Geometry check sheet. Reference: the model listing, model coordinates, mm. A direction names the side the tool comes from. Coordinates: 2 decimals unless noted, no trailing zeros. Loops run counter-clockwise (first coordinate to the right, second up) from the corner with the lowest first, then second, coordinate; pieces in that order, holes last.
from build123d import *

# Parameters (mm, degrees)
F1_DEPTH = 25.4
F3_D     = 5.1054
F4_R     = 6.35
F5_DEPTH = 12.7
F6_W     = 69.85
F6_H     = 12.7381
F7_DEPTH = 9.525
F9_D     = 6.7564
F10_R    = 4.7625


with BuildPart() as f1:
    # F0 (on Top) → F1 (new body)
    with BuildSketch(Plane.XY):
        with BuildLine():
            Line((0, 12.7), (0, 0))
            Line((0, 0), (127, 0))
            Line((127, 0), (127, 25.4))
            Line((127, 25.4), (63.5, 25.4))
            ThreePointArc((63.5, 25.4), (32.3787739113, 15.9061304434), (0, 12.7))
        make_face()
    extrude(amount=F1_DEPTH)

    # F3 (through all)
    with Locations(Plane.XZ):
        with Locations((25.4, 12.7), (82.55, 12.7)):
            Hole(F3_D / 2)

    # F4 (on face) → F5 (cut)
    with BuildSketch(Plane(origin=(0, 25.4, 0), x_dir=(-1, 0, 0), z_dir=(0, 1, 0))):
        with Locations((-25.4, 12.7)):
            Circle(F4_R)
    extrude(amount=-F5_DEPTH, mode=Mode.SUBTRACT)

    # F6 (on face) → F7 (cut)
    with BuildSketch(Plane.XY.offset(25.4)):
        with Locations((92.075, 12.71905)):
            Rectangle(F6_W, F6_H)
    extrude(amount=-F7_DEPTH, mode=Mode.SUBTRACT)

    # F9 (through all)
    with Locations(Plane.XY.offset(25.4)):
        with Locations((73.025, 12.71905), (111.125, 12.71905)):
            Hole(F9_D / 2)

    # F10
    f10_edges = [f1.edges().sort_by_distance(p)[0] for p in [
        (57.15, 19.0881, 20.6375),
        (57.15, 6.35, 20.6375),
    ]]
    fillet(f10_edges, radius=F10_R)


solid = f1.part
1) Section check D-D on y = 17.25. Record the cut outline in (x, z) (3 decimals).
Data:
outline: (38.493, 0) - (127, 0) - (127, 15.875) - (58.154, 15.875) - (58.154, 25.4) - (38.493, 25.4) - close; hole circle Ø5.105 at (82.55, 12.7)
2) Section check C-C on z = 3.25. Record the cut outline in (x, y) (3 decimals), and give its area (3 significant figures).
Data:
outline: (0, 0) - (127, 0) - (127, 25.4) - (63.5, 25.4) arc R165.1 cw to (0, 12.7) - close; hole circle Ø6.756 at (73.025, 12.719); hole circle Ø6.756 at (111.125, 12.719)
area: 2,610 mm2
3) Access from +Z, -Z, +X, -X, +Y, -Y to the whole of each face (thin tool, end or side, straight path). Record for faces 1 (the cylindrical face through (31.744, 13.92, 12.979)), 2 (the cylindrical face through (58.51, 7.78, 20.57)), 3 (the flat face through (77, 10, 0)).
Data:
face 1: +Y
face 2: +Z, +X
face 3: -Z, +X, -X, +Y, -Y
4) Mould release check, pull along Y, two halves, no side actions. Record for faces 4 (the flat face through (25, 12.7, 10)), 5 (the flat face through (63, 0, 13)), 6 (the flat face through (94, 19.088, 21)), 7 (the cylindrical face through (27.95, 6.44, 12.81)): +Y half, -Y half, draft (parallel to the pull), parting line (faces both ways), or undercut.
Data:
face 4: +Y half
face 5: -Y half
face 6: undercut
face 7: draft
5) Section check A-A on x = 82.55. Record the cut outline in (y, z) (3 decimals).
Data:
outline: (0, 0) - (25.4, 0) - (25.4, 10.147) - (0, 10.147) - close; (0, 15.253) - (25.4, 15.253) - (25.4, 25.4) - (19.088, 25.4) - (19.088, 15.875) - (6.35, 15.875) - (6.35, 25.4) - (0, 25.4) - close
6) Material ranges on probe 1 along X at (y, z) = (4.75, 12.75); probe 2 along Z at (x, y) = (25.4, 13.9); probe 3 along Y at (x, z) = (94.5, 23.25), recorded low to high.
Data:
probe 1: x = 0 to 22.85, 27.95 to 80, 85.1 to 127
probe 2: z = 0 to 6.35, 19.05 to 25.4
probe 3: y = 0 to 6.35, 19.09 to 25.4
7) Depth check by flat-ended pin: pin 1 (6 mm diameter, centred on x = 42, z = 15, fed in from +Y); pin 2 (3.5 mm diameter, centred on y = 12.5, z = 21, fed in from +X); pin 3 (11 mm diameter, centred on x = 111.12, y = 12.72, fed in from +Z) (3 decimals). Enter the tip coordinate at first touch or a pass-through.
Data:
pin 1: stops at y = 18.95
pin 2: stops at x = 57.16
pin 3: stops at z = 15.875
8) Section check B-B on z = 12.7. Record the cut outline in (x, y) (3 decimals), and give its area (3 significant figures).
Data:
outline: (0, 0) - (22.847, 0) - (22.847, 12.7) - (19.05, 12.7) - (19.05, 13.803) arc R165.1 cw to (0, 12.7) - close; (27.953, 0) - (79.997, 0) - (79.997, 25.4) - (63.5, 25.4) arc R165.1 cw to (31.75, 15.782) - (31.75, 12.7) - (27.953, 12.7) - close; (85.103, 0) - (127, 0) - (127, 25.4) - (85.103, 25.4) - close; hole circle Ø6.756 at (73.025, 12.719); hole circle Ø6.756 at (111.125, 12.719)
area: 2,390 mm2
